Model file for the job. Use its own axes, mm. Give positions to 0.01 mm unless a question says otherwise; leave off trailing zeros. Loops run counter-clockwise (first coordinate to the right, second up) from the corner with the lowest first, then second, coordinate; pieces in that order, holes last. Notation, with made-up numbers: (26, -27) -> (54, -27) arc R6 cw to (54, -20) -> close; hole circle Ø7 at (31.25, 79.5). An arc over 180 degrees is marked (long way). Use CSV: the item, a comma, the result in double quotes. Start each with the question number.
(1) Cut at D-D on z = 15. Write the cut outline in (x, y), then the cut area to 3 significant figures.
(2) Cut at A-A on z = 31.5. Write the cut outline in (x, y).
(3) Drill centre lines: probe 1 along Z at (x, y) = (47.5, 1.45); probe 2 along Z at (x, y) = (22, 0.65); probe 3 along X at (y, z) = (1.75, 46). Where is each one in solid material? Low to high.
(4) Cut at B-B on x = 47.5. Write the cut outline in (y, z), then the cut area to 3 significant figures.
(5) Flat gauge pins, fed straight in: pin 1 (2 mm diameter, centred on x = -19, z = 58.5, fed in from -Y); pin 2 (1 mm diameter, centred on y = 1.5, z = 41.5, fed in from -X). Where does each tip first touch, or does it go through?
(6) Cut at C-C on x = 28.5. Write the cut outline in (y, z).
from build123d import *

# Parameters (mm, degrees)
SKETCH_1_R          = 2
EXTRUDE_1_DEPTH     = 2
SKETCH_3_W          = 66
SKETCH_3_H          = 63
CUT_EXTRUDE_1_DEPTH = 94.21614667
FILLET_1_R          = 1
SKETCH_4_W          = 66
SKETCH_4_H          = 5
SKETCH_4_W_2        = 5
SKETCH_4_H_2        = 63
EXTRUDE_1_2_DEPTH   = 2


with BuildPart() as part:
    # 草图1 → Extrude 1 (new body)
    with BuildSketch(Plane(origin=(0, 0, 0), x_dir=(1, 0, 0), z_dir=(0, 1, 0))):
        Polygon((-52.5, -39), (-52.5, -3), (-39, -3), (-39, 0), (39, 0), (39, -3), (52.5, -3), (52.5, -39), (39, -39), (39, -77), (-39, -77), (-39, -39), align=None)
        with Locations(Location((-47.5, -8, 0), (0, 0, 270))):
            Circle(SKETCH_1_R, mode=Mode.SUBTRACT)
        with Locations(Location((-47.5, -31.5, 0), (0, 0, 270))):
            Circle(SKETCH_1_R, mode=Mode.SUBTRACT)
        with Locations(Location((47.5, -31.5, 0), (0, 0, 90))):
            Circle(SKETCH_1_R, mode=Mode.SUBTRACT)
        with Locations(Location((47.5, -8, 0), (0, 0, 90))):
            Circle(SKETCH_1_R, mode=Mode.SUBTRACT)
    extrude(amount=EXTRUDE_1_DEPTH)

    # 草图3 → 切除-拉伸1 (cut, through all)
    with BuildSketch(Plane(origin=(0, 2, 0), x_dir=(1, 0, 0), z_dir=(0, 1, 0))):
        with Locations((0, -39.5)):
            Rectangle(SKETCH_3_W, SKETCH_3_H)
    extrude(amount=-CUT_EXTRUDE_1_DEPTH, mode=Mode.SUBTRACT)

    # 圆角1
    fillet_1_edges = [part.edges().sort_by_distance(p)[0] for p in [
        (-52.5, 1, 39),
        (-52.5, 1, 3),
        (-39, 1, 3),
        (-39, 1, 0),
        (39, 1, 0),
        (39, 1, 3),
        (52.5, 1, 3),
        (52.5, 1, 39),
        (39, 1, 39),
        (39, 1, 77),
        (-39, 1, 77),
        (-39, 1, 39),
    ]]
    fillet(fillet_1_edges, radius=FILLET_1_R)

    # 草图4 → Extrude 1 2 (add)
    with BuildSketch(Plane(origin=(0, 2, 0), x_dir=(1, 0, 0), z_dir=(0, 1, 0))):
        with Locations((0, -23)):
            Rectangle(SKETCH_4_W, SKETCH_4_H)
        with Locations((0, -56)):
            Rectangle(SKETCH_4_W, SKETCH_4_H)
        with Locations((-18, -39.5)):
            Rectangle(SKETCH_4_W_2, SKETCH_4_H_2)
        with Locations((18, -39.5)):
            Rectangle(SKETCH_4_W_2, SKETCH_4_H_2)
    extrude(amount=-EXTRUDE_1_2_DEPTH)


solid = part.part
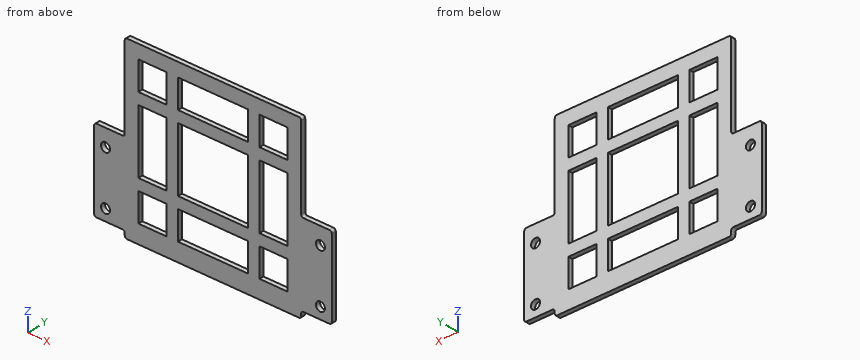
Check result:
1,outline,"(-52.5, 0) -> (-33, 0) -> (-33, 2) -> (-52.5, 2) -> close; (-20.5, 0) -> (-15.5, 0) -> (-15.5, 2) -> (-20.5, 2) -> close; (15.5, 0) -> (20.5, 0) -> (20.5, 2) -> (15.5, 2) -> close; (33, 0) -> (52.5, 0) -> (52.5, 2) -> (33, 2) -> close"
1,area,"98.0 mm²"
2,outline,"(-52.5, 0) -> (-49.5, 0) -> (-49.5, 2) -> (-52.5, 2) -> close; (-45.5, 0) -> (-33, 0) -> (-33, 2) -> (-45.5, 2) -> close; (-20.5, 0) -> (-15.5, 0) -> (-15.5, 2) -> (-20.5, 2) -> close; (15.5, 0) -> (20.5, 0) -> (20.5, 2) -> (15.5, 2) -> close; (33, 0) -> (45.5, 0) -> (45.5, 2) -> (33, 2) -> close; (49.5, 0) -> (52.5, 0) -> (52.5, 2) -> (49.5, 2) -> close"
3,probe 1,"3 to 6, 10 to 29.5, 33.5 to 39"
3,probe 2,"0 to 8, 20.5 to 25.5, 53.5 to 58.5, 71 to 77"
3,probe 3,"-39 to -33, -20.5 to -15.5, 15.5 to 20.5, 33 to 39"
4,outline,"(0, 3) -> (2, 3) -> (2, 6) -> (0, 6) -> close; (0, 10) -> (2, 10) -> (2, 29.5) -> (0, 29.5) -> close; (0, 33.5) -> (2, 33.5) -> (2, 39) -> (0, 39) -> close"
4,area,"56.0 mm²"
5,pin 1,"y = 0"
5,pin 2,"x = -39"
6,outline,"(0, 0) -> (2, 0) -> (2, 8) -> (0, 8) -> close; (0, 20.5) -> (2, 20.5) -> (2, 25.5) -> (0, 25.5) -> close; (0, 53.5) -> (2, 53.5) -> (2, 58.5) -> (0, 58.5) -> close; (0, 71) -> (2, 71) -> (2, 77) -> (0, 77) -> close"
